from build123d import *

# Parameters (mm, degrees)
SKETCH2_R           = 22.5
BOSS_EXTRUDE3_DEPTH = 25
SKETCH6_W           = 45
SKETCH6_H           = 22.5
BOSS_EXTRUDE4_DEPTH = 25
SKETCH4_R           = 20
CUT_EXTRUDE1_DEPTH  = 20
SKETCH5_R           = 2.5
CUT_EXTRUDE2_DEPTH  = 5
SKETCH7_R           = 5
CUT_EXTRUDE6_DEPTH  = 46
SKETCH9_R           = 5
SKETCH9_R_2         = 2.5
BOSS_EXTRUDE5_DEPTH = 2
SKETCH14_W          = 15
SKETCH14_H          = 5
CUT_EXTRUDE8_DEPTH  = 46.0000001
SKETCH15_W          = 25
SKETCH15_H          = 5
BOSS_EXTRUDE6_DEPTH = 37.5
SKETCH16_W          = 25
SKETCH16_H          = 5
BOSS_EXTRUDE7_DEPTH = 37.5
SKETCH19_W          = 50
SKETCH19_H          = 50
CUT_EXTRUDE9_DEPTH  = 20
BOSS_EXTRUDE8_DEPTH = 3
BOSS_EXTRUDE9_DEPTH = 3
SKETCH22_R          = 21
CUT_EXTRUDE10_DEPTH = 21.0000001
FILLET2_R           = 5


with BuildPart() as part:
    # Sketch2 → Boss-Extrude3 (new body)
    with BuildSketch(Plane.XY):
        Circle(SKETCH2_R)
    extrude(amount=BOSS_EXTRUDE3_DEPTH)

    # Sketch6 → Boss-Extrude4 (add)
    with BuildSketch(Plane.XY):
        with Locations((0, -11.25)):
            Rectangle(SKETCH6_W, SKETCH6_H)
    extrude(amount=BOSS_EXTRUDE4_DEPTH)

    # Sketch4 → Cut-Extrude1 (cut)
    with BuildSketch(Plane.XY.offset(25)):
        Circle(SKETCH4_R)
    extrude(amount=-CUT_EXTRUDE1_DEPTH, mode=Mode.SUBTRACT)

    # Sketch5 → Cut-Extrude2 (cut)
    with BuildSketch(Plane(origin=(0, 0, 0), x_dir=(-1, 0, 0), z_dir=(0, 0, -1))):
        Circle(SKETCH5_R)
    extrude(amount=-CUT_EXTRUDE2_DEPTH, mode=Mode.SUBTRACT)

    # Sketch7 → Cut-Extrude6 (cut, through all)
    with BuildSketch(Plane.XZ.offset(22.5)):
        with Locations((-10, 12.5)):
            Circle(SKETCH7_R)
        with Locations((10, 12.5)):
            Circle(SKETCH7_R)
    extrude(amount=-CUT_EXTRUDE6_DEPTH, mode=Mode.SUBTRACT)

    # Sketch9 → Boss-Extrude5 (add)
    with BuildSketch(Plane.XZ.offset(22.5)):
        with Locations((-10, 12.5)):
            Circle(SKETCH9_R)
        with Locations((-10, 12.5)):
            Circle(SKETCH9_R_2, mode=Mode.SUBTRACT)
        with Locations((10, 12.5)):
            Circle(SKETCH9_R)
        with Locations((10, 12.5)):
            Circle(SKETCH9_R_2, mode=Mode.SUBTRACT)
    extrude(amount=-BOSS_EXTRUDE5_DEPTH)

    # Sketch14 → Cut-Extrude8 (cut, through all)
    with BuildSketch(Plane(origin=(22.5, 0, 0), x_dir=(0, 0, -1), z_dir=(1, 0, 0))):
        with Locations((-12.5, 0)):
            Rectangle(SKETCH14_W, SKETCH14_H)
    extrude(amount=-CUT_EXTRUDE8_DEPTH, mode=Mode.SUBTRACT)

    # Sketch15 → Boss-Extrude6 (add)
    with BuildSketch(Plane.ZY.offset(22.5)):
        with Locations((12.5, -20)):
            Rectangle(SKETCH15_W, SKETCH15_H)
    extrude(amount=BOSS_EXTRUDE6_DEPTH)

    # Sketch16 → Boss-Extrude7 (add)
    with BuildSketch(Plane(origin=(22.5, 0, 0), x_dir=(0, 0, -1), z_dir=(1, 0, 0))):
        with Locations((-12.5, -20)):
            Rectangle(SKETCH16_W, SKETCH16_H)
    extrude(amount=BOSS_EXTRUDE7_DEPTH)

    # Sketch19 → Cut-Extrude9 (cut)
    with BuildSketch(Plane.XY.offset(25)):
        with Locations((2.5, 7.5)):
            Rectangle(SKETCH19_W, SKETCH19_H)
    extrude(amount=-CUT_EXTRUDE9_DEPTH, mode=Mode.SUBTRACT)

    # Sketch24 → Boss-Extrude8 (add)
    with BuildSketch(Plane.ZY.offset(22.5)):
        Polygon((5, 0), (5, -17.5), (25, -17.5), align=None)
    extrude(amount=-BOSS_EXTRUDE8_DEPTH)

    # Sketch25 → Boss-Extrude9 (add)
    with BuildSketch(Plane(origin=(22.5, 0, 0), x_dir=(0, 0, -1), z_dir=(1, 0, 0))):
        Polygon((-5, 0), (-25, -17.5), (-5, -17.5), align=None)
    extrude(amount=-BOSS_EXTRUDE9_DEPTH)

    # Sketch22 → Cut-Extrude10 (cut, through all)
    with BuildSketch(Plane.XY.offset(5)):
        Circle(SKETCH22_R)
    extrude(amount=CUT_EXTRUDE10_DEPTH, mode=Mode.SUBTRACT)

    # Fillet2
    fillet2_edges = [part.edges().sort_by_distance(p)[0] for p in [
        (22.5, -17.5, 12.5),
        (-22.5, -17.5, 12.5),
    ]]
    fillet(fillet2_edges, radius=FILLET2_R)


solid = part.part
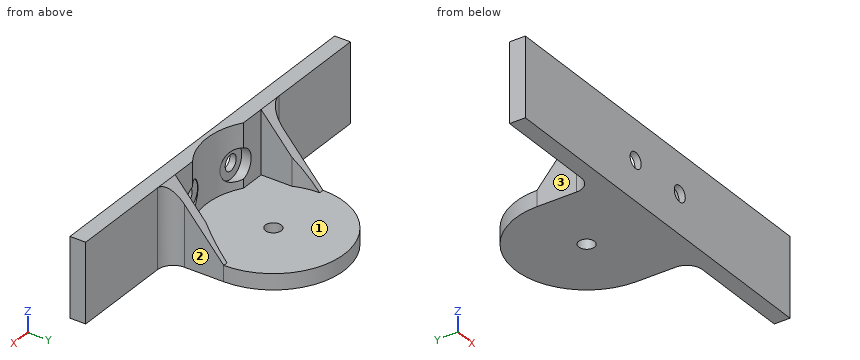
The listing builds one solid part. Answer for the finished solid, in the listing's coordinates (mm). Face numbers are marked on the shaded views. A direction names the side the tool comes from. Round coordinates to 2 decimals unless told otherwise and drop trailing zeros. Order: outer loops, then holes, each group sorted by start corner. A loop starts at its lowest first (then second) coordinate and runs counter-clockwise, first axis right, second up. Notation, with made-up numbers: (76, -32) -> (131, -32) arc R33 ccw to (131, 4) -> close; hole circle Ø9 at (79, 73.25). An arc over 180 degrees is marked (long way). One line per item, written item: value.
Item 1: Given P1, Ø8, axis at x = 19.5, y = 12.5, coming from the -Z side; P2, Ø6, axis at x = -3.5, y = 16.5, coming from the +Z side; P3, Ø10.5, axis at y = -10, z = 13.5, coming from the +X side; P4, Ø13, axis at x = 10, z = 12.5, coming from the +Y side, each flat-ended and moving along its own axis, determine where each tip first touches the part or whether it passes through.
Taken from the geometry:
P1: stops at z = 0
P2: stops at z = 5
P3: stops at x = 23.32
P4: stops at y = -17.5
Item 2: Find section A-A, the plane x = 9. Give the vertices of the cut face in (y, z), then the cut area to 3 significant figures.
Taken from the geometry:
outline: (-22.5, 0) -> (20.62, 0) -> (20.62, 5) -> (-18.97, 5) -> (-18.97, 7.6) -> (-20.5, 7.6) -> (-20.5, 10.21) -> (-22.5, 10.21) -> close; (-22.5, 14.79) -> (-20.5, 14.79) -> (-20.5, 17.4) -> (-18.97, 17.4) -> (-18.97, 25) -> (-22.5, 25) -> close
area: 262 mm2
Item 3: Straight lines are drawn through the part: L1, parallel to Z at x = 10, y = -19; L2, parallel to X at y = -12, z = 9; L3, parallel to Z at x = 10, y = -21.6. For each, find the intervals that lie inside material, in ascending order.
Taken from the geometry:
L1: z = 0 to 7.5, 17.5 to 25
L2: x = -22.5 to -19.5, 19.5 to 22.5
L3: z = 0 to 10, 15 to 25
Item 4: Find section B-B, the plane z = 21.75. Give the vertices of the cut face in (x, y), then the cut area to 3 significant figures.
Taken from the geometry:
outline: (-60, -22.5) -> (60, -22.5) -> (60, -17.5) -> (27.5, -17.5) arc R5 cw to (22.99, -14.66) -> (19.5, -14.66) -> (19.5, -17.5) -> (11.61, -17.5) arc R21 cw to (-11.61, -17.5) -> (-19.5, -17.5) -> (-19.5, -14.66) -> (-22.99, -14.66) arc R5 cw to (-27.5, -17.5) -> (-60, -17.5) -> close
area: 572 mm2
Item 5: Find section D-D, the plane x = -33.5. Give the vertices of the cut face in (y, z).
Taken from the geometry:
outline: (-22.5, 0) -> (-17.5, 0) -> (-17.5, 25) -> (-22.5, 25) -> close
Item 6: For the marked faces 1, 2 and 3, determine the directions among +Z, -Z, +X, -X, +Y, -Y from which every point of the face is accessible in a straight line to the end or side of a thin tool.
Taken from the geometry:
face 1: +Z, +Y
face 2: +Z, -Z, +X, +Y
face 3: +Z, -Z, -X, +Y
Item 7: Find section C-C, the plane y = -9.5. Give the vertices of the cut face in (x, z), then the cut area to 3 significant figures.
Taken from the geometry:
outline: (-22.5, 0) -> (22.5, 0) -> (22.5, 15.86) -> (19.5, 15.86) -> (19.5, 5) -> (-19.5, 5) -> (-19.5, 15.86) -> (-22.5, 15.86) -> close
area: 290 mm2
